Verification items for the finished model (mm, model axes). A direction names the side the tool comes from. Give positions to 0.01 mm unless a question says otherwise; leave off trailing zeros. Order: outer loops, then holes, each group sorted by start corner. A loop starts at its lowest first (then second) coordinate and runs counter-clockwise, first axis right, second up. Notation, with made-up numbers: (48, 13.25) - (82, 13.25) arc R18 ccw to (82, 30.25) - close; hole circle Ø7 at (3, 53). An arc over 180 degrees is marked (long way). Answer as a JSON object with one key per item and string values.
Autodesk Inventor part; units mm, degrees
ref_plane "Work Plane1" through (0, 50, 0) normal (0, 1, 0) x (-1, 0, 0)
ref_plane "Work Plane2" through (0, 0, -79) normal (0, 0, 1) x (1, 0, 0)
ref_plane "Work Plane3" through (-40, 45, 40) normal (0, -1, 0) x (1, 0, 0)
sketch "Sketch2" plane through (0, 0, 0) normal (0, 1, 0) x (-1, 0, 0)
  line L0 (15, 15) -> (-15, 15)
  line L1 (-15, -15) -> (15, -15)
  line L2 (15, 4.5) -> (8, 4.5)
  line L3 (8, 4.5) -> (8, -4.5)
  line L4 (8, -4.5) -> (15, -4.5)
  line L5 (-15, 4.5) -> (-8, 4.5)
  line L6 (-8, 4.5) -> (-8, -4.5)
  line L7 (-8, -4.5) -> (-15, -4.5)
  line L8 (15, -15) -> (15, -4.5)
  line L9 (15, 4.5) -> (15, 15)
  line L10 (-15, 15) -> (-15, 4.5)
  line L11 (-15, -4.5) -> (-15, -15)
  point P0 (0, 0)
  dimension "d18" = 9
  dimension "d19" = 7
  dimension "d21" = 16
  dimension "d22" = 30
  dimension "d23" = 15
  dimension "d24" = 4.5
  dimension "d25" = 8
sketch "Sketch6" plane through (0, 0, 0) normal (0, 0, 1) x (1, 0, 0)
  arc A0 (0, 0) -> (-110, 190.5256) centre (-220, 0) ccw
  line L0 (-220, 0) -> (-110, 190.5256) construction
  line L1 (-220, 0) -> (0, 0) construction
  dimension "d41" = 220
  dimension "d42" = 60
  dimension "d43" = 220
  dimension "d44" = 0
sweep "Sweep2" add profiles "Sketch2" path "Sketch6"
sketch "Sketch7" plane through (-102.5, 203.516, 4.5) normal (-0.8660254, 0.5, 0) x (0, 0, 1)
  line L0 (-16.5, -3) -> (-12, -3)
  line L1 (-12, -3) -> (-12, -10)
  line L2 (-12, -10) -> (3, -10)
  line L3 (3, -10) -> (3, -3)
  line L4 (3, -3) -> (7.5, -3)
  line L5 (7.5, -3) -> (7.5, -27)
  line L6 (7.5, -27) -> (3, -27)
  line L7 (3, -27) -> (3, -20)
  line L8 (3, -20) -> (-12, -20)
  line L9 (-12, -20) -> (-12, -27)
  line L10 (-12, -27) -> (-16.5, -27)
  line L11 (-16.5, -27) -> (-16.5, -3)
  line L12 (-19.5, 0) -> (-19.5, -30)
  line L13 (-9, -7) -> (-9, 0)
  line L14 (0, 0) -> (0, -7)
  line L15 (10.5, -30) -> (10.5, 0)
  line L16 (-19.5, -30) -> (-9, -30)
  line L17 (-9, 0) -> (-19.5, 0)
  line L18 (0, -30) -> (10.5, -30)
  line L19 (-9, -23) -> (0, -23)
  line L20 (0, -7) -> (-9, -7)
  point P0 (-4.5, -125)
  point P1 (-14.25, 0)
  dimension "d47" = 3
  dimension "d48" = 3
  dimension "d49" = 3
  dimension "d50" = 3
  dimension "d51" = 3
  dimension "d52" = 3
  dimension "d53" = 3
  dimension "d54" = 3
  dimension "d55" = 3
extrude "Extrusion3" add sketch "Sketch7" along normal blind 10
sketch "Sketch8" plane through (-116, 180.1333, -12) normal (0, 0, -1) x (-0.8660254, 0.5, 0)
  circle A0 centre (5, 12) radius 2
  line L0 (0, 0) -> (10, 0)
  line L1 (10, 24) -> (10, 0)
  point P0 (-190.5256, -98)
  dimension "d58" = 4
  dimension "d59" = 12
  dimension "d60" = 5
extrude "Extrusion4" cut sketch "Sketch8" against normal through all
sketch "Sketch9" plane through (0, 0, 0) normal (0, 1, 0) x (-1, 0, 0)
  line L0 (-40, 40) -> (40, 40)
  line L1 (40, 40) -> (40, -40)
  line L2 (40, -40) -> (-40, -40)
  line L3 (-40, -40) -> (-40, 40)
  point P0 (0, 0)
  dimension "d63" = 80
  dimension "d64" = 80
  dimension "d65" = 40
  dimension "d66" = 40
ref_plane "Work Plane1" through (0, 50, 0) normal (0, 1, 0) x (-1, 0, 0)
sketch "Sketch10" plane through (0, 50, 0) normal (0, 1, 0) x (-1, 0, 0)
  line L0 (-9.6, 15) -> (21.4, 15)
  line L1 (21.4, 15) -> (21.4, -15)
  line L2 (21.4, -15) -> (-9.6, -15)
  line L3 (-9.6, -15) -> (-9.6, 15)
  point P0 (0, 0)
  dimension "d68" = 30
  dimension "d69" = 9.6
  dimension "d70" = 15
  dimension "d71" = 31
loft "Loft1" add profiles "Sketch9", "Sketch10"
ref_plane "Work Plane2" through (0, 0, -79) normal (0, 0, 1) x (1, 0, 0)
sketch "Sketch11" plane through (0, 0, -79) normal (0, 0, 1) x (1, 0, 0)
  line L0 (50, -5) -> (-129.034, -5)
  line L1 (-129.034, -5) -> (-129.034, 135)
  line L2 (-129.034, 135) -> (-90, 202.6089)
  line L3 (-90, 202.6089) -> (50, 95)
  line L4 (50, -5) -> (50, 95)
  point P0 (0, 0)
  dimension "d77" = 100
  dimension "d79" = 140
  dimension "d80" = 67.6089
  dimension "d81" = 140
  dimension "d82" = 150
  dimension "d83" = 50
  dimension "d86" = 5
extrude "Extrusion5" [suppressed]
sketch "Sketch12" plane through (-40, 0, 40) normal (0, -1, 0) x (1, 0, 0)
  line L0 (70, -70) -> (10, -70)
  line L1 (10, -70) -> (10, -10)
  line L2 (10, -10) -> (70, -10)
  line L3 (70, -10) -> (70, -70)
  line L4 (0, 0) -> (0, -80)
  line L5 (0, -80) -> (80, -80)
  line L6 (80, -80) -> (80, 0)
  line L7 (80, 0) -> (0, 0)
  point P0 (40, -40)
  dimension "d87" = 10
  dimension "d88" = 10
  dimension "d89" = 10
  dimension "d90" = 10
ref_plane "Work Plane3" through (-40, 45, 40) normal (0, -1, 0) x (1, 0, 0)
sketch "Sketch14" plane through (-40, 45, 40) normal (0, -1, 0) x (1, 0, 0)
  line L0 (40.5, -40.5) -> (39.5, -40.5)
  line L1 (39.5, -40.5) -> (39.5, -39.5)
  line L2 (39.5, -39.5) -> (40.5, -39.5)
  line L3 (40.5, -39.5) -> (40.5, -40.5)
  line L4 (80, 0) -> (0, 0)
  line L5 (0, 0) -> (0, -80)
  point P0 (40, -40)
  point P1 (0, -40)
  dimension "d95" = 1
  dimension "d96" = 1
  dimension "d97" = 39.5
  dimension "d98" = 39.5
loft "Loft2" cut profiles "Sketch12", "Sketch14" contours L0 L1 L2 L3 / all
ref_plane "Work Plane4" through (9.6, 50, -45) normal (0, 0, -1) x (-1, 0, 0)
sketch "Sketch15" plane through (9.6, 50, -45) normal (0, 0, -1) x (-1, 0, 0)
  line L0 (-151.4512, 170) -> (229.6, 170)
  line L1 (229.6, 170) -> (229.6, -50)
  line L2 (229.6, -50) -> (-151.4512, 170)
  line L3 (0, 0) -> (7.15, 0) construction
  line L4 (229.6, -50) -> (9.6, -50) construction
  dimension "d105" = 220
  dimension "d107" = 0
  dimension "d108" = 30
  dimension "d109" = 220
extrude "Extrusion6" cut sketch "Sketch15" against normal through all
sketch "Sketch16" plane through (-42.4648, 102.5, 15) normal (-0.5, 0.8660254, 0) x (0.8660254, 0.5, 0)
  line L0 (27, 27) -> (27, 22.5)
  line L1 (27, 22.5) -> (20, 22.5)
  line L2 (20, 22.5) -> (20, 7.5)
  line L3 (18.8407, 0) -> (18.8407, 10.5)
  line L4 (20, 7.5) -> (27, 7.5)
  line L5 (27, 7.5) -> (27, 3)
  line L6 (27, 3) -> (3, 3)
  line L7 (3, 3) -> (3, 7.5)
  line L8 (3, 7.5) -> (10, 7.5)
  line L9 (10, 7.5) -> (10, 22.5)
  line L10 (10, 22.5) -> (3, 22.5)
  line L11 (3, 22.5) -> (3, 27)
  line L12 (3, 27) -> (27, 27)
  line L13 (30, 30) -> (30, 19.5)
  line L14 (30, 19.5) -> (23, 19.5)
  line L15 (0, 30) -> (30, 30)
  line L16 (23, 19.5) -> (23, 10.5)
  line L17 (23, 10.5) -> (30, 10.5)
  line L18 (30, 0) -> (0, 0)
  line L19 (7, 10.5) -> (7, 19.5)
  line L20 (0, 0) -> (0, 10.5)
  line L21 (0, 19.5) -> (0, 30)
  point P0 (-14.4744, 15)
  dimension "d112" = 3
  dimension "d113" = 3
  dimension "d114" = 3
  dimension "d115" = 3
  dimension "d116" = 3
  dimension "d117" = 3
  dimension "d118" = 3
  dimension "d119" = 3
  dimension "d120" = 3
extrude "Extrusion7" add sketch "Sketch16" along normal blind 10
properties part number "LightRail_endSection"
(1) Access from +Z, -Z, +X, -X, +Y, -Y to the whole of each face (thin tool, end or side, straight path). Record for faces 1 (the flat face through (-14, 77, 15)), 2 (the flat face through (-26, 77, 4.5)), 3 (the flat face through (-25, 119, -7.5)).
Computed values:
{"face 1": "+Z, +X, -X, +Y", "face 2": "-X", "face 3": "+Y"}
(2) Gauge pin test, flat ends, axial feed: pin 1 Ø12 at (x, y) = (-25, 120.5) entering from +Z; pin 2 Ø12 at (y, z) = (44.5, -28.5) entering from +X; pin 3 Ø0.5 at (x, z) = (0, 0) entering from -Y; pin 4 Ø12 at (x, y) = (-40.5, 112) entering from -Z. Record the tip position at first contact, or that the pin passes through.
Computed values:
{"pin 1": "stops at z = 12", "pin 2": "passes through", "pin 3": "stops at y = 45", "pin 4": "stops at z = -12"}
(3) Release check for a two-part mould opening along Z. For faces 4 (the flat face through (-35.43, 106.56, -0.21)), 5 (the flat face through (-15, 76, -15)), 6 (the flat face through (-4, 83, 4.5)), 7 (the flat face through (-42.33, 108.27, -9.72)) record: pulls with the +Z half, pulls with the -Z half, needs draft (parallel to the pull), parting line crosses it, or undercut.
Computed values:
{"face 4": "undercut", "face 5": "pulls with the -Z half", "face 6": "undercut", "face 7": "needs draft"}
(4) Section check A-A (y = 94). Record the cut outline in (x, z), then the cut area to 3 significant figures.
Computed values:
{"outline": "(-37.82, -15) - (-4.62, -15) - (-4.62, -4.5) - (-12.28, -4.5) - (-12.28, 4.5) - (-4.62, 4.5) - (-4.62, 15) - (-37.82, 15) - (-37.82, 4.5) - (-29.98, 4.5) - (-29.98, -4.5) - (-37.82, -4.5) - close", "area": "857 mm²"}
(5) Material ranges on line 1 along Z through (x, y) = (-29.5, 92.5); line 2 along Z through (x, y) = (16, 16.5); line 3 along Z through (x, y) = (-30.5, 116.5), recorded low to high. Write a range as [from, to].
Computed values:
{"line 1": "z = [-15, -4.5], [4.5, 15]", "line 2": "z = [-31.75, -19.18], [19.18, 31.75]", "line 3": "z = [-12, 12]"}
